Autodesk Inventor part; units mm, degrees
ref_plane "YZ Plane" through (0, 0, 0) normal (1, 0, 0) x (0, 1, 0)
ref_plane "XZ Plane" through (0, 0, 0) normal (0, 1, 0) x (-1, 0, 0)
ref_plane "XY Plane" through (0, 0, 0) normal (0, 0, 1) x (1, 0, 0)
sketch "unten" plane through (0, 0, 0) normal (0, 0, 1) x (1, 0, 0)
  line L0 (0, 0) -> (130, 0)
  line L1 (130, 0) -> (130, -50)
  line L2 (130, -50) -> (0, -50)
  line L3 (0, -50) -> (0, 0)
  line L4 (23.5, -7) -> (52.1715, -7)
  line L5 (58, -12.8285) -> (58, -41.5)
  line L6 (27.8285, -43) -> (56.5, -43)
  line L7 (22, -8.5) -> (22, -37.1715)
  arc A0 (23.5, -7) -> (22, -8.5) centre (23.5, -8.5) ccw
  circle A1 centre (23, -42) radius 1
  circle A2 centre (57, -8) radius 1
  arc A3 (56.5, -43) -> (58, -41.5) centre (56.5, -41.5) ccw
  line L8 (61.9906, -8.5458) -> (71.0184, -8.5458) construction
  line L9 (53.5857, -7.5858) -> (57.4142, -11.4143)
  line L10 (57.2091, -11.2092) -> (62.6234, -11.2092) construction
  arc A4 (58, -12.8285) -> (57.4142, -11.4143) centre (56, -12.8285) ccw
  arc A5 (53.5857, -7.5858) -> (52.1715, -7) centre (52.1715, -9) ccw
  line L11 (22.5858, -38.5857) -> (26.4143, -42.4142)
  line L12 (26.3083, -42.3082) -> (31.7226, -42.3082) construction
  arc A6 (22, -37.1715) -> (22.5858, -38.5857) centre (24, -37.1715) ccw
  arc A7 (26.4143, -42.4142) -> (27.8285, -43) centre (27.8285, -41) ccw
  line L13 (130, -9.5) -> (130, -40.5)
  line L14 (130, -50) -> (130, 0)
  line L15 (130, 0) -> (130, -50)
  point P0 (33.5, -8.5)
  dimension "d0" = 130
  dimension "d1" = 50
  dimension "d15" = 1.5
  dimension "d18" = 2
  dimension "d21" = 2
  dimension "d24" = 1.5
  dimension "d29" = 45
  dimension "d31" = 2
  dimension "d32" = 45
  dimension "d34" = 2
  dimension "d51" = 7
  dimension "d52" = 7
  dimension "d53" = 36
  dimension "d55" = 8
  dimension "d56" = 1
  dimension "d57" = 1
  dimension "d58" = 1
  dimension "d59" = 2.1214
  dimension "d60" = 22
  dimension "d61" = 1.5
  dimension "d62" = 1.5
  dimension "d63" = 2.1214
  dimension "d64" = 1.5
  dimension "d65" = 1.5
extrude "Extrusion1" add sketch "unten" along normal blind 10
sketch "Sketch2" plane through (0, 0, 10) normal (0, 0, 1) x (1, 0, 0)
  line L0 (114, -9.5) -> (130, -9.5)
  line L1 (130, -50) -> (130, 0)
  line L2 (130, 0) -> (0, 0)
  line L3 (130, -9.5) -> (130, 0)
  line L4 (130, 0) -> (0, 0)
  line L5 (130, 0) -> (100, 0)
  line L6 (100, 0) -> (100, -50)
  line L7 (0, -50) -> (130, -50)
  line L8 (130, -50) -> (130, -40.5)
  line L9 (130, -40.5) -> (114, -40.5)
  line L10 (114, -12.5) -> (114, -37.5)
  arc A0 (114, -9.5) -> (114, -12.5) centre (114, -11) ccw
  arc A1 (114, -37.5) -> (114, -40.5) centre (114, -39) ccw
  dimension "d69" = 16
  dimension "d70" = 9.5
  dimension "d71" = 30
  dimension "d72" = 9.5
  dimension "d73" = 16
  dimension "d74" = 16
  dimension "d75" = 16
  dimension "d77" = 1.5
  dimension "d78" = 3
  dimension "d80" = 1.5
extrude "Extrusion2" add sketch "Sketch2" along normal blind 4 contours A0 L10 A1 L9 L1 L7 L6 L2 L0
sketch "Sketch3" plane through (0, 0, 10) normal (0, 0, 1) x (1, 0, 0)
  line L0 (100, -50) -> (100, 0)
  line L1 (0, -4) -> (100, -4)
  line L2 (100, -4) -> (100, -46)
  line L3 (100, -46) -> (0, -46)
  line L4 (0, -46) -> (0, -4)
  line L5 (100, 0) -> (0, 0)
  line L6 (0, -50) -> (100, -50)
  dimension "d83" = 4
  dimension "d84" = 4
extrude "Extrusion3" cut sketch "Sketch3" against normal blind 2
sketch "Sketch4" plane through (0, 0, 8) normal (0, 0, 1) x (1, 0, 0)
  line L0 (61, -4) -> (19, -4)
  line L1 (19, -4) -> (19, -46)
  line L2 (19, -46) -> (61, -46)
  line L3 (61, -46) -> (61, -4)
  line L4 (22, -8.5) -> (22, -37.1715)
  line L5 (27.8285, -43) -> (56.5, -43)
  point P0 (0, 0)
  dimension "d87" = 42
  dimension "d88" = 42
  dimension "d89" = 3
  dimension "d90" = 3
extrude "Extrusion4" cut sketch "Sketch4" against normal blind 5
sketch "Sketch5" plane through (0, 0, 0) normal (0, 0, -1) x (-1, 0, 0)
  line L0 (-19, -46) -> (-19, -4)
  line L1 (-61, -4) -> (-61, -46)
  line L2 (-19, -46) -> (-61, -46)
  line L3 (-61, -46) -> (-61, -4)
  line L4 (-61, -4) -> (-19, -4)
  line L5 (-19, -4) -> (-19, -46)
  point P0 (0, 0)
extrude "Extrusion5" cut sketch "Sketch5" against normal blind 1.4
fillet "Fillet1" radius 6 1 edges at (0, -25, 0)
sketch "Sketch6" plane through (0, 0, 0) normal (0, 0, -1) x (-1, 0, 0)
  line L0 (-6, -50) -> (-130, -50)
  line L1 (-130, 0) -> (-6, 0)
  line L2 (-130, -50) -> (-130, 0)
  point P0 (0, 0)
  point P1 (-122.5, -35.5)
  point P2 (-122.5, -14.5)
  dimension "d96" = 14.5
  dimension "d97" = 14.5
  dimension "d98" = 7.5
  dimension "d99" = 7.5
hole "Hole1" at (122.5, -35.5, 0) at (122.5, -14.5, 0) direction (0, 0, 1) diameter 4.5 end through all counterbore diameter 8 counterbore depth 3
sketch "Sketch7" plane through (0, 0, 0) normal (0, 0, -1) x (-1, 0, 0)
  line L0 (-130, 0) -> (-6, 0)
  line L1 (-100, -4) -> (-100, -46)
  point P0 (0, 0)
  point P1 (-90, -25)
  dimension "d119" = 25
  dimension "d120" = 10
hole "Hole2" at (90, -25, 0) direction (0, 0, 1) diameter 4.5 end through all counterbore diameter 8 counterbore depth 3
hole "Hole4" at (25, -50, 6) direction (0, 1, 0) diameter 2 end through all
pattern_linear "Rectangular Pattern1" count 4 spacing 10 along (1, 0, 0) of "Hole4"
sketch "Sketch10" plane through (0, 0, 10) normal (0, 0, 1) x (1, 0, 0)
  line L0 (130, -9.5) -> (114, -9.5)
  line L1 (130, -9.5) -> (114, -9.5)
  arc A0 (114, -9.5) -> (114, -12.5) centre (114, -11) ccw
  arc A1 (114, -12.5) -> (114, -12.5) centre (114, -11) ccw
  arc A2 (114, -37.5) -> (114, -40.5) centre (114, -39) ccw
  line L2 (114, -12.5) -> (114, -37.5)
  arc A3 (114, -37.5) -> (114, -40.5) centre (114, -39) ccw
  line L3 (114, -40.5) -> (130, -40.5)
  line L4 (114, -40.5) -> (130, -40.5)
  line L5 (130, -50) -> (130, 0)
  line L6 (130, -40.5) -> (130, -9.5)
  line L7 (130, -9.5) -> (130, -40.5)
  point P0 (0, 0)
extrude "Extrusion6" cut sketch "Sketch10" against normal blind 5
sketch "Sketch11" plane through (0, -50, 10) normal (0, -1, 0) x (1, 0, 0)
  circle A0 centre (25, -4) radius 1
  line L0 (100, 0) -> (0, 0)
  line L1 (24, -4) -> (26, -4)
  line L2 (26, -4) -> (26, 0)
  line L3 (26, 0) -> (24, 0)
  line L4 (24, 0) -> (24, -4)
  point P0 (0, -10)
extrude "Extrusion7" cut sketch "Sketch11" against normal through all contours L1 A0 | A0 L4 L0 L2 picked at (25.0402, -3.6691)
pattern_linear "Rectangular Pattern2" count 4 spacing 10 along (1, 0, 0) of "Extrusion7"
properties part number "TNS_Greiferbacke_MA_Jun_T1"
Check sheet for the modelled part. Datum: model origin and axes. Units: mm. A direction names the side the tool comes from. Give positions to 0.01 mm unless a question says otherwise; leave off trailing zeros. Order: outer loops, then holes, each group sorted by start corner. A loop starts at its lowest first (then second) coordinate and runs counter-clockwise, first axis right, second up. Notation, with made-up numbers: (49.25, 8) -> (90.25, 8) arc R33 ccw to (90.25, 47) -> close; hole circle Ø2 at (-30.5, 71.25). An arc over 180 degrees is marked (long way). Use CSV: the item, a comma, the result in double quotes. Start each with the question number.
1) Sectioned sample at B-B, the plane x = 73. Record the boundary of the cut face in (y, z).
2) Mould release check, pull along Y, two halves, no side actions. Record for faces 1 (the face through (111, -25, 14)), 2 (the face through (64, 0, 5)), 3 (the face through (124.2, -12.8, 3)): released by +Y, released by -Y, zero draft, split by the parting line, or undercut.
3) Material ranges on line 1 (X direction, y = -3, z = 6.75); line 2 (Y direction, x = 122.5, z = 3.6); line 3 (Y direction, x = 59, z = 6.75), recorded low to high. Write a range as from..to.
4) Go/stop test with flat-tipped pins: P1, Ø15, axis at x = 6, y = -26.5, coming from the +Z side; P2, Ø1.2, axis at x = 38.5, y = -49, coming from the +Z side; P3, Ø5, axis at x = 60, y = -32.5, coming from the -Z side; P4, Ø2, axis at y = -7.5, z = 3, coming from the -X side. Record where each tip stops, or that it passes through.
5) Sectioned sample at A-A, the plane y = -14.5. Give the number of separate pieces and of enclosed holes in the cut face, plus the area to 3 significant figures.
6) Set-up check for faces 4 (the face through (19, -25, 6)), 5 (the face through (118.534, -36.021, 1.521)), 6 (the face through (46, -2, 8)): record each of +Z, -Z, +X, -X, +Y, -Y from which the full face is reachable in a straight line by a thin tool's end or side.
Recorded:
1,outline,"(-50, 0) -> (0, 0) -> (0, 10) -> (-4, 10) -> (-4, 8) -> (-46, 8) -> (-46, 10) -> (-50, 10) -> close"
2,face 1,"zero draft"
2,face 2,"released by +Y"
2,face 3,"undercut"
3,line 1,"0..24, 26..34, 36..44, 46..54, 56..130"
3,line 2,"-50..-37.75, -33.25..-16.75, -12.25..0"
3,line 3,"-50..-46, -4..0"
4,P1,"z = 8"
4,P2,"z = 10"
4,P3,"z = 0"
4,P4,"x = 0.34"
5,separate pieces,"3"
5,enclosed holes,"0"
5,area,"709 mm2"
6,face 4,"+Z"
6,face 5,"-Z"
6,face 6,"+Z, +Y, -Y"
